Geometry: final body of the model. Coordinates: model frame, mm. A direction names the side the tool comes from. Round coordinates to 2 decimals unless told otherwise and drop trailing zeros. Loops run counter-clockwise (first coordinate to the right, second up) from the corner with the lowest first, then second, coordinate; pieces in that order, holes last. Notation, with made-up numbers: (53.5, 59.5) -> (72.5, 59.5) arc R34 ccw to (72.5, 89.5) -> close; hole circle Ø3 at (21.5, 62). An arc over 180 degrees is marked (long way). Answer in a Markdown table with one row per item.
Autodesk Inventor part; units mm, degrees
ref_plane "YZ Plane" through (0, 0, 0) normal (1, 0, 0) x (0, 1, 0)
ref_plane "XZ Plane" through (0, 0, 0) normal (0, 1, 0) x (-1, 0, 0)
ref_plane "XY Plane" through (0, 0, 0) normal (0, 0, 1) x (1, 0, 0)
sketch "Sketch1" plane through (0, 0, 0) normal (0, 1, 0) x (-1, 0, 0)
  point P0 (0, 0)
sketch "Sketch2" plane through (0, 0, 0) normal (0, 1, 0) x (-1, 0, 0)
  line L0 (0, 0) -> (3, 0)
  line L1 (3, 0) -> (3, -40)
  line L2 (3, -40) -> (0, -40)
  line L3 (0, -40) -> (0, 0)
  line L4 (0, -40) -> (-3, -40)
  line L5 (-3, -40) -> (-3, -35)
  line L6 (-3, -35) -> (0, -35)
  line L7 (0, -35) -> (0, -40)
  point P0 (0, -35)
  dimension "d0" = 3
  dimension "d1" = 40
  dimension "d4" = 3
  dimension "d5" = 5
extrude "Extrusion1" add sketch "Sketch2" along normal blind 1.2
fillet "Fillet1" radius 2 4 edges at (0, 0.6, -35) (3, 0.6, -35) (3, 0.6, -40) (-3, 0.6, -40)
properties part number "MoveableBarRound"
Item 1: Set-up query: faces 1 (the flat face through (0, 1, -17)), 2 (the cylindrical face through (-2.4, 0.61, -39.43)). Return all of +Z, -Z, +X, -X, +Y, -Y with unobstructed straight access to the full face (end or side cutting, diameter ignored); none if empty.
Ans:
| item | result |
|---|---|
| face 1 | +Z, +X, +Y, -Y |
| face 2 | -Z, -X, +Y, -Y |
Item 2: Section query A-A, the plane z = -21. Output: boundary loops of the cut face in (x, y), and give its area (3 significant figures).
Ans:
| item | result |
|---|---|
| outline | (-3, 0) -> (0, 0) -> (0, 1.2) -> (-3, 1.2) -> close |
| area | 3.60 mm2 |
Item 3: Section query B-B, the plane x = -2.5. Output: boundary loops of the cut face in (y, z), and give its area (3 significant figures).
Ans:
| item | result |
|---|---|
| outline | (0, -39.32) -> (1.2, -39.32) -> (1.2, 0) -> (0, 0) -> close |
| area | 47.2 mm2 |
Item 4: Ray query, L1, parallel to X at y = 0.4, z = -21; L2, parallel to Z at x = 2.25, y = 0.8; L3, parallel to Z at x = 2.5, y = 0.9. Return the intervals inside material, ascending.
Ans:
| item | result |
|---|---|
| L1 | -3 to 0 |
| L2 | -39.56 to -35.31 |
| L3 | -39.32 to -35.55 |
